from build123d import *

# Parameters (mm, degrees)
SKETCH2_W          = 457.2
SKETCH2_H          = 50.8
BASE_DEPTH         = 6
CUT_EXTRUDE1_REACH = 8
SKETCH3_W          = 6
SKETCH3_H          = 16.933333334
SKETCH3_H_2        = 11.733333334
CUT_EXTRUDE2_REACH = 8
SKETCH4_W          = 10.18
SKETCH4_H          = 6
CUT_EXTRUDE3_REACH = 8


with BuildPart() as part:
    # Sketch2 → Base (new body)
    with BuildSketch(Plane(origin=(0, 0, 0), x_dir=(1, 0, 0), z_dir=(0, 1, 0))):
        with Locations((228.6, 25.4)):
            Rectangle(SKETCH2_W, SKETCH2_H)
    extrude(amount=BASE_DEPTH)

    # Sketch3 → Cut-Extrude1 (cut, up to next)
    with BuildSketch(Plane(origin=(0, 6, 0), x_dir=(1, 0, 0), z_dir=(0, 1, 0)), mode=Mode.PRIVATE) as cut_extrude1_sk1:
        with Locations((438.74, 25.4)):
            Rectangle(SKETCH3_W, SKETCH3_H)
    cut_extrude1_tool1 = extrude(cut_extrude1_sk1.sketch, amount=-CUT_EXTRUDE1_REACH, mode=Mode.PRIVATE) & part.part
    add(cut_extrude1_tool1.solids().sort_by_distance((438.74, 6, -25.4))[0], mode=Mode.SUBTRACT)
    # Sketch3 → Cut-Extrude1 (cut, up to next)
    with BuildSketch(Plane(origin=(0, 6, 0), x_dir=(1, 0, 0), z_dir=(0, 1, 0)), mode=Mode.PRIVATE) as cut_extrude1_sk2:
        with Locations((27.54, 25.4)):
            Rectangle(SKETCH3_W, SKETCH3_H_2)
    cut_extrude1_tool2 = extrude(cut_extrude1_sk2.sketch, amount=-CUT_EXTRUDE1_REACH, mode=Mode.PRIVATE) & part.part
    add(cut_extrude1_tool2.solids().sort_by_distance((27.54, 6, -25.4))[0], mode=Mode.SUBTRACT)

    # Sketch4 → Cut-Extrude2 (cut, up to next)
    with BuildSketch(Plane(origin=(0, 6, 0), x_dir=(1, 0, 0), z_dir=(0, 1, 0)), mode=Mode.PRIVATE) as cut_extrude2_sk1:
        with Locations((15.27, 4.8)):
            Rectangle(SKETCH4_W, SKETCH4_H)
    cut_extrude2_tool1 = extrude(cut_extrude2_sk1.sketch, amount=-CUT_EXTRUDE2_REACH, mode=Mode.PRIVATE) & part.part
    add(cut_extrude2_tool1.solids().sort_by_distance((15.27, 6, -4.8))[0], mode=Mode.SUBTRACT)
    # Sketch4 → Cut-Extrude2 (cut, up to next)
    with BuildSketch(Plane(origin=(0, 6, 0), x_dir=(1, 0, 0), z_dir=(0, 1, 0)), mode=Mode.PRIVATE) as cut_extrude2_sk2:
        with Locations((15.27, 46)):
            Rectangle(SKETCH4_W, SKETCH4_H)
    cut_extrude2_tool2 = extrude(cut_extrude2_sk2.sketch, amount=-CUT_EXTRUDE2_REACH, mode=Mode.PRIVATE) & part.part
    add(cut_extrude2_tool2.solids().sort_by_distance((15.27, 6, -46))[0], mode=Mode.SUBTRACT)

    # Sketch5 → Cut-Extrude3 (cut, up to next)
    with BuildSketch(Plane(origin=(0, 6, 0), x_dir=(1, 0, 0), z_dir=(0, 1, 0)), mode=Mode.PRIVATE) as cut_extrude3_sk1:
        Polygon((214.894666784, 33.866666667), (242.305333216, 33.866666667), (410.34, 33.866666667), (410.34, 16.933333333), (242.305333216, 16.933333333), (214.894666784, 16.933333333), (55.94, 16.933333333), (55.94, 33.866666667), align=None)
    cut_extrude3_tool1 = extrude(cut_extrude3_sk1.sketch, amount=-CUT_EXTRUDE3_REACH, mode=Mode.PRIVATE) & part.part
    add(cut_extrude3_tool1.solids().sort_by_distance((233.14, 6, -25.4))[0], mode=Mode.SUBTRACT)


solid = part.part
Geometry: final body of the model. Coordinates: model frame, mm. Coordinates: 2 decimals unless noted, no trailing zeros. Order: outer loops, then holes, each group sorted by start corner. A loop starts at its lowest first (then second) coordinate and runs counter-clockwise, first axis right, second up.
(1) Section query A-A (x = 195.5). Return the cut outline in (y, z), plus the area to 3 significant figures.
(2) Material intervals for probe 1 along X at (y, z) = (0.4, -25); probe 2 along X at (y, z) = (4.85, -48.5); probe 3 along Z at (x, y) = (72.5, 2.3), sorted ascending.
(3) Section query B-B (y = 3.65). Return the cut outline in (x, z), plus the area to 3 significant figures.
Solution:
1. outline: (0, -50.8) - (6, -50.8) - (6, -33.87) - (0, -33.87) - close; (0, -16.93) - (6, -16.93) - (6, 0) - (0, 0) - close
1. area: 203 mm2
2. probe 1: x = 0 to 24.54, 30.54 to 55.94, 410.34 to 435.74, 441.74 to 457.2
2. probe 2: x = 0 to 10.18, 20.36 to 457.2
2. probe 3: z = -50.8 to -33.87, -16.93 to 0
3. outline: (0, -50.8) - (457.2, -50.8) - (457.2, 0) - (0, 0) - close; hole (10.18, -49) - (20.36, -49) - (20.36, -43) - (10.18, -43) - close; hole (10.18, -7.8) - (20.36, -7.8) - (20.36, -1.8) - (10.18, -1.8) - close; hole (24.54, -31.27) - (30.54, -31.27) - (30.54, -19.53) - (24.54, -19.53) - close; hole (55.94, -33.87) - (410.34, -33.87) - (410.34, -16.93) - (55.94, -16.93) - close; hole (435.74, -33.87) - (441.74, -33.87) - (441.74, -16.93) - (435.74, -16.93) - close
3. area: 16,900 mm2
